Geometry check sheet. Reference: the model listing, model coordinates, mm. Round coordinates to 2 decimals unless told otherwise and drop trailing zeros. Loops run counter-clockwise (first coordinate to the right, second up) from the corner with the lowest first, then second, coordinate; pieces in that order, holes last. Notation, with made-up numbers: (-30, 25) -> (-25, 25) arc R13 cw to (-25, 45) -> close; hole circle Ø11 at (45, 43.25). An arc over 180 degrees is marked (long way). Use one line per item in the form item = value.
from build123d import *

# Parameters (mm, degrees)
BOSS_EXTRUDE3_DEPTH      = 50
BOSS_EXTRUDE3_DEPTH_BACK = 15


with BuildPart() as part:
    # Sphere Sketch → Sphere (revolve)
    with BuildSketch(Plane(origin=(0, 0, 0), x_dir=(0, 0, -1), z_dir=(1, 0, 0))):
        with BuildLine():
            Line((-587.274308735, 273.648124971), (-552.558139535, 257.471673071))
            Line((-552.558139535, 257.471673071), (-495, 230.651707126))
            ThreePointArc((-495, 230.651707126), (55.906074852, 543.230817236), (531.601551916, 125))
            Line((531.601551916, 125), (593.41568586, 139.534883721))
            Line((593.41568586, 139.534883721), (618.141339438, 145.348837209))
            Line((618.141339438, 145.348837209), (568.384355354, 220.343787272))
            ThreePointArc((568.384355354, 220.343787272), (89.800502747, 602.949442082), (-479.506339183, 376.411783401))
            Line((-479.506339183, 376.411783401), (-533.692189105, 315.721145663))
            ThreePointArc((-533.692189105, 315.721145663), (-539.321048901, 312.550143885), (-545.714010445, 313.482537358))
            Line((-545.714010445, 313.482537358), (-559.670433417, 320.673382776))
            ThreePointArc((-559.670433417, 320.673382776), (-561.95861772, 320.863883523), (-563.711312727, 319.380597256))
            Line((-563.711312727, 319.380597256), (-587.274308735, 273.648124971))
        make_face()
    revolve(axis=Axis((0, 0, 0), (0, 0, -1)))

    # Sketch1 → Boss-Extrude3 (add, two sides: drawn at the far end of the back side and taken through both)
    with BuildSketch(Plane(origin=(0, 296.514361113, 575.492810731), x_dir=(1, 0, 0), z_dir=(0, 0.45801563170636533, 0.8889441383532597)).offset(-BOSS_EXTRUDE3_DEPTH_BACK)):
        with BuildLine():
            Line((114.40522717, -36.492315976), (134.313589091, -36.492315976))
            Line((134.313589091, -36.492315976), (134.313589091, -15.953517695))
            ThreePointArc((134.313589091, -15.953517695), (134.020695872, -15.246410914), (133.313589091, -14.953517695))
            Line((133.313589091, -14.953517695), (114.40522717, -14.953517695))
            ThreePointArc((114.40522717, -14.953517695), (113.698120389, -15.246410914), (113.40522717, -15.953517695))
            Line((113.40522717, -15.953517695), (113.40522717, -35.492315976))
            ThreePointArc((113.40522717, -35.492315976), (113.698120389, -36.199422758), (114.40522717, -36.492315976))
        make_face()
    extrude(amount=BOSS_EXTRUDE3_DEPTH + BOSS_EXTRUDE3_DEPTH_BACK)


solid = part.part
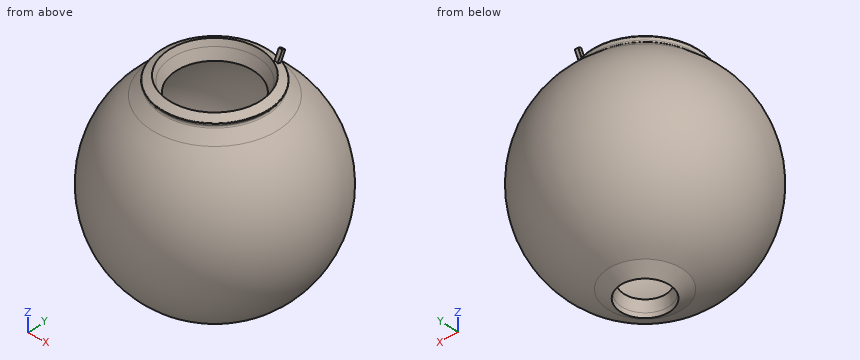
1. Material ranges on line 1 along Y through (x, z) = (73, -417); line 2 along Z through (x, y) = (-153, -194); line 3 along X through (y, z) = (265.5, 111), recorded low to high.
Return value:
line_1 = -438.63 to -344.97, 344.97 to 438.63
line_2 = -557.29 to -487.01, 487.01 to 530.24
line_3 = -537.4 to -464.13, 464.13 to 537.4
2. Section check B-B (x = 459.5). Record the boundary of the cut face in (y, z).
Return value:
outline = circle Ø801.18 at (0, 0); hole circle Ø590.2 at (0, 0)
3. Gauge pin test, flat ends, axial feed: pin 1 (3 mm diameter, centred on x = 310, z = 327.5, fed in from +Y); pin 2 (22.5 mm diameter, centred on y = 287.5, z = 607.5, fed in from -X); pin 3 (5 mm diameter, centred on x = 253.5, y = 301, fed in from -Z). Record the tip position at first contact, or that the pin passes through.
Return value:
pin_1 = 411.83
pin_2 = 113.41
pin_3 = -467.66
4. Section check A-A (y = 394.5). Record the boundary of the cut face in (x, z).
Return value:
outline = circle Ø929.48 at (0, 0); hole circle Ø755.23 at (0, 0)
